Autodesk Inventor part; units mm, degrees
ref_plane "YZ Plane" through (0, 0, 0) normal (1, 0, 0) x (0, 1, 0)
ref_plane "XZ Plane" through (0, 0, 0) normal (0, 1, 0) x (-1, 0, 0)
ref_plane "XY Plane" through (0, 0, 0) normal (0, 0, 1) x (1, 0, 0)
sketch "Sketch1" plane through (0, 0, 0) normal (0, 0, 1) x (1, 0, 0)
  line L0 (0, 5.815) -> (0, 4)
  line L1 (4, 4) -> (25, 4)
  line L2 (25, 4) -> (25, 0)
  line L3 (25, 0) -> (-0.6001, 0)
  line L4 (-3.0501, 0) -> (32.65, 0)
  line L5 (-0.6001, 0) -> (-0.6001, 5.815)
  line L6 (-0.6001, 5.815) -> (0, 5.815)
  line L7 (4, 4) -> (3.2331, 4)
  line L8 (3.2331, 4) -> (0, 4)
  line L9 (0, -0.344) -> (0, 4.472)
  dimension "d0" = 25
  dimension "d1" = 21
  dimension "d2" = 8
  dimension "d9" = 0.6001
  dimension "d10" = 11.63
  dimension "d13" = 0.7669
  dimension "d14" = 8
revolve "Body" add sketch "Sketch1" angle 360 about axis through (25, 0, 0) along (-1, 0, 0)
sketch "Sketch2" plane through (-0.6001, 0, 0) normal (-1, 0, 0) x (0, 0, 1)
  line L0 (0, 7.5056) -> (6.5, 3.7528)
  line L1 (6.5, 3.7528) -> (6.5, -3.7528)
  line L2 (6.5, -3.7528) -> (0, -7.5056)
  line L3 (0, -7.5056) -> (-6.5, -3.7528)
  line L4 (-6.5, -3.7528) -> (-6.5, 3.7528)
  line L5 (-6.5, 3.7528) -> (0, 7.5056)
  point P0 (0, 0)
  point P1 (0, 0)
  dimension "d11" = 13
extrude "Head" add sketch "Sketch2" along normal blind 4.7
sketch "Sketch4" plane through (0, 0, 0) normal (0, 0, 1) x (1, 0, 0)
  line L0 (-5.3001, 6.5) -> (-5.3001, 7.5056)
  line L1 (-5.3001, 7.5056) -> (-4.7195, 7.5056)
  line L2 (-4.7195, 7.5056) -> (-5.3001, 6.5)
  line L3 (-3.8001, 0) -> (0.3999, 0)
  line L4 (-0.6001, 7.5056) -> (-5.3001, 7.5056)
  line L5 (-5.3001, 3.7528) -> (-5.3001, 7.5056)
  dimension "d5" = 30
  dimension "d19" = 13
revolve "Chamfer1" cut sketch "Sketch4" angle 360 about axis through (-10, 0, 0) along (1, 0, 0)
thread "Thread"
chamfer "Chamfer2" distance 0.7668 distance2 0.7669 1 edges at (25, -4, 0) measured on face at (25, 0.998, -0.8842)
equation "\"d0\" = NLG"
equation "\"d1\" = GEL"
equation "\"d2\" = GD"
equation "\"d10\" = SD2"
equation "\"d14\" = BDM"
equation "\"d11\" = SW"
equation "\"d3\" = KOH - SD"
equation "\"d5\" = ANG1"
equation "\"d19\" = SW0"
equation "\"d15\" = GEL"
equation "\"d6\" = -0.5 * SPD + 0.5 * GD"
equation "\"NLG\" = 25"
equation "\"GD\" = NND"
equation "\"BDM\" = NND"
equation "\"KOH\" = 5.3"
equation "\"GEL\" = 21"
equation "\"SW\" = 13"
equation "\"SW0\" = SW"
equation "\"SPD\" = NND - 1.2269 * TPU"
equation "\"SD2\" = 11.63"
equation "\"SD\" = 0.6"
equation "\"ANG1\" = 30deg"
equation "\"GAL\" = 0.61345 * TPU"
equation "\"GUL\" = 0.61345 * TPU"
equation "\"RR\" = 0.4"
equation "\"d20\" = -NLG"
equation "\"TOA\" = 30deg"
equation "\"PTC\" = TPU"
equation "\"GD1\" = THREADDIA - 1.2269 * TPU"
equation "\"TPU\" = 1.25"
equation "\"THREADDIA\" = 8"
equation "\"SDH\" = SD2"
equation "\"E0\" = 15.015"
equation "\"NND\" = 8"
equation "\"SDHG\" = 4"
properties part number "ISO 4017 - M8 x 25" material "Steel, Mild"
The model under review builds one solid part; all positions refer to its coordinate system, in mm. A direction names the side the tool comes from. Give positions to 0.01 mm unless a question says otherwise; leave off trailing zeros. Write each loop counter-clockwise with the first axis right and the second up, starting at its lowest first coordinate (ties: lowest second). Pieces come first, ordered by that corner, then holes. Notation, with made-up numbers: (71.25, 34) -> (120.25, 34) arc R36 ccw to (120.25, 73) -> close; hole circle Ø5 at (-37.5, 34). An arc over 180 degrees is marked (long way). Answer in a Markdown table with one row per item.
1) Tool access review of faces 1 (the flat face through (-2.92, -5.66, -3.2)), 2 (the flat face through (0, 1.2, -4)): name each direction out of +Z, -Z, +X, -X, +Y, -Y from which nothing blocks a thin tool from reaching the whole face with its end or side.
Worked answers:
| item | result |
|---|---|
| face 1 | -Z, +X, -X, -Y |
| face 2 | +X |
2) For L1, parallel to X at y = 2, z = -3.75; L2, parallel to Y at x = 18, z = 0; L3, parallel to X at y = 5.5, z = 2.5, list the stretches that pass through material, from the lowest coordinate up. Write a range as [from, to].
Worked answers:
| item | result |
|---|---|
| L1 | [-5.3, 0] |
| L2 | [-4, 4] |
| L3 | [-5.3, -0.6] |
3) Add section A-A on x = 22. State the section outline as (y, z) points.
Worked answers:
| item | result |
|---|---|
| outline | circle Ø8 at (0, 0) |
4) Clearance check with flat-ended pins moving along their axes: P1, Ø2, axis at y = -5, z = -4.5, coming from the +X side; P2, Ø3, axis at x = 3.5, z = -1.5, coming from the +Y side; P3, Ø5, axis at x = 8.5, z = -2.5, coming from the -Y side. State where each tip first meets the part, or that it passes through.
Worked answers:
| item | result |
|---|---|
| P1 | x = 0 |
| P2 | y = 4 |
| P3 | y = -4 |
